```python
from build123d import *

# Parameters (mm, degrees)
PAD009_DEPTH    = 2.8
FILLET004_R     = 0.4
SKETCH025_W     = 12.7
SKETCH025_H     = 1.6
POCKET014_DEPTH = 2.801
SKETCH026_R     = 0.25
POCKET015_DEPTH = 2.801


with BuildPart() as part:
    # Sketch009 (on Face6 of ShapeBinder008) → Pad009 (new body)
    with BuildSketch(Plane.XZ.offset(60.388718)):
        with BuildLine():
            Line((37.8, 3.127675), (37.8, 0.327675))
            Line((37.8, 0.327675), (23.8, 0.327675))
            ThreePointArc((23.8, 0.327675), (23.4, -0.072325), (23.8, -0.472325))
            Line((23.8, -0.472325), (37.8, -0.472325))
            Line((37.8, -0.472325), (37.8, -33.872325))
            Line((37.8, -33.872325), (23.8, -33.872325))
            ThreePointArc((23.8, -33.872325), (23.4, -34.272325), (23.8, -34.672325))
            Line((23.8, -34.672325), (37.8, -34.672325))
            Line((37.8, -34.672325), (37.8, -37.472325))
            Line((37.8, -37.472325), (35.8, -38.222325))
            Line((35.8, -38.222325), (35.8, -37.472325))
            Line((35.8, -37.472325), (33, -37.472325))
            Line((33, -37.472325), (33, -39.472325))
            Line((33, -39.472325), (25.535898, -37.472325))
            Line((25.535898, -37.472325), (-25.535898, -37.472325))
            Line((-25.535898, -37.472325), (-33, -39.472325))
            Line((-33, -39.472325), (-33, -37.472325))
            Line((-33, -37.472325), (-35.8, -37.472325))
            Line((-35.8, -38.222325), (-35.8, -37.472325))
            Line((-37.8, -37.472325), (-35.8, -38.222325))
            Line((-37.8, -37.472325), (-37.8, -34.672325))
            Line((-37.8, -34.672325), (-23.8, -34.672325))
            ThreePointArc((-23.8, -34.672325), (-23.4, -34.272325), (-23.8, -33.872325))
            Line((-23.8, -33.872325), (-37.8, -33.872325))
            Line((-37.8, -33.872325), (-37.8, -0.472325))
            Line((-37.8, -0.472325), (-23.8, -0.472325))
            ThreePointArc((-23.8, -0.472325), (-23.4, -0.072325), (-23.8, 0.327675))
            Line((-23.8, 0.327675), (-37.8, 0.327675))
            Line((-37.8, 0.327675), (-37.8, 3.127675))
            Line((-37.8, 3.127675), (-35.8, 3.877675))
            Line((-35.8, 3.877675), (-35.8, 3.127675))
            Line((-35.8, 3.127675), (-33, 3.127675))
            Line((-33, 3.127675), (-33, 5.127675))
            Line((-33, 5.127675), (-25.535898, 3.127675))
            Line((-25.535898, 3.127675), (25.535898, 3.127675))
            Line((25.535898, 3.127675), (33, 5.127675))
            Line((33, 5.127675), (33, 3.127675))
            Line((33, 3.127675), (35.8, 3.127675))
            Line((35.8, 3.877675), (35.8, 3.127675))
            Line((37.8, 3.127675), (35.8, 3.877675))
        make_face()
    extrude(amount=-PAD009_DEPTH)

    # Fillet004
    fillet004_edges = [part.edges().sort_by_distance(p)[0] for p in [
        (33, -58.988718, 5.127675),
        (37.8, -58.988718, 3.127675),
        (37.8, -58.988718, 0.327675),
        (37.8, -58.988718, -0.472325),
        (37.8, -58.988718, -33.872325),
        (37.8, -58.988718, -34.672325),
        (37.8, -58.988718, -37.472325),
        (33, -58.988718, -39.472325),
        (-37.8, -58.988718, -33.872325),
        (-37.8, -58.988718, -34.672325),
        (-37.8, -58.988718, -37.472325),
        (-33, -58.988718, -39.472325),
        (-33, -58.988718, 5.127675),
        (-37.8, -58.988718, 3.127675),
        (-37.8, -58.988718, 0.327675),
        (-37.8, -58.988718, -0.472325),
    ]]
    fillet(fillet004_edges, radius=FILLET004_R)

    # Sketch025 (on Face2 of Fillet004) → Pocket014 (cut, through all)
    with BuildSketch(Plane.XZ.offset(60.388718)):
        with Locations((-19.05, -5.2)):
            Rectangle(SKETCH025_W, SKETCH025_H)
        with Locations((19.05, -5.2)):
            Rectangle(SKETCH025_W, SKETCH025_H)
    extrude(amount=-POCKET014_DEPTH, mode=Mode.SUBTRACT)

    # Sketch026 (on Face2 of Pocket014) → Pocket015 (cut, through all)
    with BuildSketch(Plane.XZ.offset(60.388718)):
        with Locations((-25.4, -4.4)):
            Circle(SKETCH026_R)
        with Locations((-12.7, -4.4)):
            Circle(SKETCH026_R)
        with Locations((-12.7, -6)):
            Circle(SKETCH026_R)
        with Locations((-25.4, -6)):
            Circle(SKETCH026_R)
        with Locations((12.7, -4.4)):
            Circle(SKETCH026_R)
        with Locations((12.7, -6)):
            Circle(SKETCH026_R)
        with Locations((25.4, -4.4)):
            Circle(SKETCH026_R)
        with Locations((25.4, -6)):
            Circle(SKETCH026_R)
    extrude(amount=-POCKET015_DEPTH, mode=Mode.SUBTRACT)


solid = part.part
```
Work out the finished part from the listing and answer in its coordinate system (mm). A direction names the side the tool comes from. Round coordinates to 2 decimals unless told otherwise and drop trailing zeros. Order: outer loops, then holes, each group sorted by start corner. A loop starts at its lowest first (then second) coordinate and runs counter-clockwise, first axis right, second up.
Q1. Given pin 1 Ø1.4 at (x, y) = (-31, -59) entering from +Z; pin 2 Ø0.8 at (x, y) = (29, -59) entering from +Z; pin 3 Ø1.4 at (x, y) = (0.5, -59) entering from -Z, each flat-ended and moving along its own axis, determine where each tip first touches the part or whether it passes through.
Solution:
pin 1: stops at z = 4.78
pin 2: stops at z = 4.16
pin 3: stops at z = -37.47
Q2. A tool of negligible diameter and unlimited length cuts with its end or side. For faces 1 (the flat face through (31, -59, -33.872)), 2 (the flat face through (34, -59, 3.128)), 3 (the flat face through (-19, -59, -6)), from which of +Z, -Z, +X, -X, +Y, -Y can it reach the whole face along a straight path? Write none if from no direction.
Solution:
face 1: +X, +Y, -Y
face 2: +Z, +Y, -Y
face 3: +Y, -Y
Q3. Find the intervals of material crossed by line 1 along Z through (x, y) = (-34, -58.45); line 2 along Z through (x, y) = (17, -58.6); line 3 along Z through (x, y) = (-26.5, -60.1), in increasing order.
Solution:
line 1: z = -37.47 to -34.67, -33.87 to -0.47, 0.33 to 3.13
line 2: z = -37.47 to -6, -4.4 to 3.13
line 3: z = -37.73 to -34.67, -33.87 to -0.47, 0.33 to 3.39
Q4. A cutting plane is placed at C-C, the plane x = -5. Determine the outline of the cut face in (y, z), then the cut area to 3 significant figures.
Solution:
outline: (-60.39, -37.47) - (-57.59, -37.47) - (-57.59, 3.13) - (-60.39, 3.13) - close
area: 114 mm2
Q5. A cutting plane is placed at A-A, the plane x = -18.5. Determine the outline of the cut face in (y, z).
Solution:
outline: (-60.39, -37.47) - (-57.59, -37.47) - (-57.59, -6) - (-60.39, -6) - close; (-60.39, -4.4) - (-57.59, -4.4) - (-57.59, 3.13) - (-60.39, 3.13) - close
Q6. A cutting plane is placed at B-B, the plane y = -58.6. Count the separate pieces of the cut face and the enclosed holes in it, then the cut area to 3 significant figures.
Solution:
separate pieces: 1
enclosed holes: 2
area: 3,010 mm2
Q7. The mould has two halves that part along Z. Classify faces 4 (the flat face through (-36.682, -59.008, -37.891)), 5 (the flat face through (-31, -59, -0.472)), 6 (the flat face through (1, -60.389, -17)), 7 (the flat face through (-31, -59, 0.328)): pulls with the +Z half, pulls with the -Z half, needs draft (parallel to the pull), parting line crosses it, or undercut.
Solution:
face 4: pulls with the -Z half
face 5: undercut
face 6: needs draft
face 7: undercut
